```python
from build123d import *

# Parameters (mm, degrees)
CROQUIS1_W              = 750
CROQUIS1_H              = 400
SALIENTE_EXTRUIR1_DEPTH = 30
CROQUIS2_W              = 720
CROQUIS2_H              = 370
CORTAR_EXTRUIR1_DEPTH   = 2
REDONDEO1_R             = 8


with BuildPart() as part:
    # Croquis1 → Saliente-Extruir1 (new body)
    with BuildSketch(Plane.XY):
        with Locations((375, 200)):
            Rectangle(CROQUIS1_W, CROQUIS1_H)
    extrude(amount=SALIENTE_EXTRUIR1_DEPTH)

    # Croquis2 → Cortar-Extruir1 (cut)
    with BuildSketch(Plane.XY.offset(30)):
        with Locations((375, 200)):
            Rectangle(CROQUIS2_W, CROQUIS2_H)
    extrude(amount=-CORTAR_EXTRUIR1_DEPTH, mode=Mode.SUBTRACT)

    # Redondeo1
    redondeo1_edges = [part.edges().sort_by_distance(p)[0] for p in [
        (0, 400, 15),
        (750, 400, 15),
        (750, 0, 15),
        (0, 0, 15),
    ]]
    fillet(redondeo1_edges, radius=REDONDEO1_R)


solid = part.part
```
For this review, take the finished solid that the model builds, in its own axes (mm). Give positions to 0.01 mm unless a question says otherwise; leave off trailing zeros. Write each loop counter-clockwise with the first axis right and the second up, starting at its lowest first coordinate (ties: lowest second). Pieces come first, ordered by that corner, then holes. Notation, with made-up numbers: M -8,-33.5 L 23,-33.5 A22 ccw 23,-18.5 Z; hole C -25,-37.5 d7. An arc over 180 degrees is marked long. Answer as a JSON object with one key per item and string values. Group by question number.
Item 1: Consider section B-B on x = 647.5. Write out the cut boundary in (y, z).
Item 2: Consider section A-A on y = 183. Write out the cut boundary in (x, z), plus the area to 3 significant figures.
Item 3: For pin 1 Ø3 at (x, y) = (369, 250.5) entering from +Z, flat-tipped, find the tip position at first contact; note if it passes through.
Item 4: For probe 1 along Z at (x, y) = (588, 153); probe 2 along X at (y, z) = (44.5, 28.25), list the stretches that pass through material, from the lowest coordinate up. Write a range as [from, to].
Item 5: Draft analysis for pull direction X (two halves, no side actions). For faces 1 (the flat face through (370, 400, 15)), 2 (the flat face through (370, 203, 28)), 3 (the flat face through (750, 197, 15)), state which applies: +X half, -X half, draft (parallel to the pull), parting line (faces both ways), or undercut.
Check result:
{
 "1": {"outline": "M 0,0 L 400,0 L 400,30 L 385,30 L 385,28 L 15,28 L 15,30 L 0,30 Z"},
 "2": {"outline": "M 0,0 L 750,0 L 750,30 L 735,30 L 735,28 L 15,28 L 15,30 L 0,30 Z", "area": "21,100 mm^2"},
 "3": {"pin 1": "stops at z = 28"},
 "4": {"probe 1": "z = [0, 28]", "probe 2": "x = [0, 15], [735, 750]"},
 "5": {"face 1": "draft", "face 2": "undercut", "face 3": "+X half"}
}
